Geometry: final body of the model. Coordinates: model frame, mm. A direction names the side the tool comes from. Give positions to 0.01 mm unless a question says otherwise; leave off trailing zeros. Loops run counter-clockwise (first coordinate to the right, second up) from the corner with the lowest first, then second, coordinate; pieces in that order, holes last. Notation, with made-up numbers: M 17,29 L 45,29 A32 ccw 45,57 Z; hole C 62,33.5 d11. An arc over 180 degrees is marked long. Put each result on its own line as item: value.
```python
from build123d import *

# Parameters (mm, degrees)
F1_DEPTH       = 25
F2_W           = 5
F2_H           = 25
F3_DEPTH       = 40
F4_R           = 5
F6_D           = 4
F6_CSINK_D     = 7
F6_CSINK_ANGLE = 90


# Not quite as in the source:
# - a feature names something its author has since deleted; it is built from what else it names


with BuildPart() as f1:
    # F0 (on Top) → F1 (new body)
    with BuildSketch(Plane.XY):
        with BuildLine():
            ThreePointArc((-14.3421743065, 17.5), (-10.0120472875, 16.123724357), (-7.2711064946, 12.5))
            Line((-7.2711064946, 12.5), (7.2711064946, 12.5))
            ThreePointArc((7.2711064946, 12.5), (10.0120472875, 16.123724357), (14.3421743065, 17.5))
            Line((14.3421743065, 17.5), (-14.3421743065, 17.5))
        make_face()
        with BuildLine():
            ThreePointArc((-7.2711064946, -12.5), (-10.0120472875, -16.123724357), (-14.3421743065, -17.5))
            Line((-14.3421743065, -17.5), (12.8716113806, -17.5))
            ThreePointArc((12.8716113806, -17.5), (8.5414843617, -16.123724357), (5.8005435687, -12.5))
            Line((5.8005435687, -12.5), (-7.2711064946, -12.5))
        make_face()
        with BuildLine():
            ThreePointArc((14.3421743065, 17.5), (10.0120472875, 16.123724357), (7.2711064946, 12.5))
            Line((7.2711064946, 12.5), (14.3421743065, 12.5))
            ThreePointArc((14.3421743065, 12.5), (16.1099412594, 11.767766953), (16.8421743065, 10))
            ThreePointArc((16.8421743065, 10), (16.1099412594, 8.232233047), (14.3421743065, 7.5))
            Line((14.3421743065, 7.5), (8.5, 7.5))
            ThreePointArc((8.5, 7.5), (12.7884854356, 6.1529580422), (15.5364989199, 2.5957047116))
            ThreePointArc((15.5364989199, 2.5957047116), (20.052140795, 5.1372556412), (21.8421743065, 10))
            ThreePointArc((21.8421743065, 10), (19.6454751654, 15.3033008589), (14.3421743065, 17.5))
        make_face()
        with BuildLine():
            ThreePointArc((-14.3421743065, 7.5), (-16.8421743065, 10), (-14.3421743065, 12.5))
            Line((-14.3421743065, 12.5), (-7.2711064946, 12.5))
            ThreePointArc((-7.2711064946, 12.5), (-10.0120472875, 16.123724357), (-14.3421743065, 17.5))
            ThreePointArc((-14.3421743065, 17.5), (-21.8182098422, 10.5990765131), (-15.5364989199, 2.5957047116))
            ThreePointArc((-15.5364989199, 2.5957047116), (-12.7884854356, 6.1529580422), (-8.5, 7.5))
            Line((-8.5, 7.5), (-14.3421743065, 7.5))
        make_face()
        with BuildLine():
            ThreePointArc((-7.3056753865, 7.4042952884), (-7.9009234869, 7.4760355357), (-8.5, 7.5))
            ThreePointArc((-8.5, 7.5), (-12.7884854356, 6.1529580422), (-15.5364989199, 2.5957047116))
            ThreePointArc((-15.5364989199, 2.5957047116), (-14.9412508196, 2.5239644643), (-14.3421743065, 2.5))
            ThreePointArc((-14.3421743065, 2.5), (-10.0536888708, 3.8470419578), (-7.3056753865, 7.4042952884))
        make_face()
        with BuildLine():
            ThreePointArc((-1, 0), (-2.7900335114, 4.8627443588), (-7.3056753865, 7.4042952884))
            ThreePointArc((-7.3056753865, 7.4042952884), (-10.0536888708, 3.8470419578), (-14.3421743065, 2.5))
            Line((-14.3421743065, 2.5), (-8.5, 2.5))
            ThreePointArc((-8.5, 2.5), (-6.732233047, 1.767766953), (-6, 0))
            ThreePointArc((-6, 0), (-6.732233047, -1.767766953), (-8.5, -2.5))
            Line((-8.5, -2.5), (-14.3421743065, -2.5))
            ThreePointArc((-14.3421743065, -2.5), (-10.0536888708, -3.8470419578), (-7.3056753865, -7.4042952884))
            ThreePointArc((-7.3056753865, -7.4042952884), (-2.7900335114, -4.8627443588), (-1, 0))
        make_face()
        with BuildLine():
            ThreePointArc((-14.3421743065, -2.5), (-14.9412508196, -2.5239644643), (-15.5364989199, -2.5957047116))
            ThreePointArc((-15.5364989199, -2.5957047116), (-12.7884854356, -6.1529580422), (-8.5, -7.5))
            ThreePointArc((-8.5, -7.5), (-7.9009234869, -7.4760355357), (-7.3056753865, -7.4042952884))
            ThreePointArc((-7.3056753865, -7.4042952884), (-10.0536888708, -3.8470419578), (-14.3421743065, -2.5))
        make_face()
        with BuildLine():
            ThreePointArc((12.8716113806, -2.5), (8.7359797123, -3.7432795568), (5.9714803927, -7.0609198123))
            ThreePointArc((5.9714803927, -7.0609198123), (7.2168200812, -7.3894146789), (8.5, -7.5))
            ThreePointArc((8.5, -7.5), (12.6356316683, -6.2567204432), (15.4001309879, -2.9390801877))
            ThreePointArc((15.4001309879, -2.9390801877), (14.1547912994, -2.6105853211), (12.8716113806, -2.5))
        make_face()
        with BuildLine():
            ThreePointArc((8.5, 7.5), (7.9009234869, 7.4760355357), (7.3056753865, 7.4042952884))
            ThreePointArc((7.3056753865, 7.4042952884), (9.8321935715, 4.0074985381), (13.7956134511, 2.5199417628))
            ThreePointArc((13.7956134511, 2.5199417628), (14.6682639838, 2.5070923186), (15.5364989199, 2.5957047116))
            ThreePointArc((15.5364989199, 2.5957047116), (12.7884854356, 6.1529580422), (8.5, 7.5))
        make_face()
        with BuildLine():
            ThreePointArc((13.7956134511, 2.5199417628), (9.8321935715, 4.0074985381), (7.3056753865, 7.4042952884))
            ThreePointArc((7.3056753865, 7.4042952884), (1.0317000428, 0.6888365189), (5.9714803927, -7.0609198123))
            ThreePointArc((5.9714803927, -7.0609198123), (8.7359797123, -3.7432795568), (12.8716113806, -2.5))
            Line((12.8716113806, -2.5), (8.5, -2.5))
            ThreePointArc((8.5, -2.5), (6.0000044235, -0.0047029402), (8.4905941362, 2.4999823059))
            Line((8.4905941362, 2.4999823059), (13.7956134511, 2.5199417628))
        make_face()
        with BuildLine():
            ThreePointArc((-8.5, -7.5), (-12.7884854356, -6.1529580422), (-15.5364989199, -2.5957047116))
            ThreePointArc((-15.5364989199, -2.5957047116), (-21.8182098422, -10.5990765131), (-14.3421743065, -17.5))
            ThreePointArc((-14.3421743065, -17.5), (-10.0120472875, -16.123724357), (-7.2711064946, -12.5))
            Line((-7.2711064946, -12.5), (-14.3421743065, -12.5))
            ThreePointArc((-14.3421743065, -12.5), (-16.8421743065, -10), (-14.3421743065, -7.5))
            Line((-14.3421743065, -7.5), (-8.5, -7.5))
        make_face()
        with BuildLine():
            Line((12.8716113806, -12.5), (5.8005435687, -12.5))
            ThreePointArc((5.8005435687, -12.5), (8.5414843617, -16.123724357), (12.8716113806, -17.5))
            ThreePointArc((12.8716113806, -17.5), (18.1749122395, -15.3033008589), (20.3716113806, -10))
            ThreePointArc((20.3716113806, -10), (19.0040618311, -5.6822399936), (15.4001309879, -2.9390801877))
            ThreePointArc((15.4001309879, -2.9390801877), (12.6356316683, -6.2567204432), (8.5, -7.5))
            Line((8.5, -7.5), (12.8716113806, -7.5))
            ThreePointArc((12.8716113806, -7.5), (14.6393783336, -8.232233047), (15.3716113806, -10))
            ThreePointArc((15.3716113806, -10), (14.6393783336, -11.767766953), (12.8716113806, -12.5))
        make_face()
    extrude(amount=F1_DEPTH)

    # F2 (on Right) → F3 (join, symmetric)
    with BuildSketch(Plane.YZ):
        with Locations((15, 12.5)):
            Rectangle(F2_W, F2_H)
    extrude(amount=F3_DEPTH, both=True)

    # F4
    f4_edges = [f1.edges().sort_by_distance(p)[0] for p in [
        (40, 15, 0),
        (40, 15, 25),
        (-40, 15, 25),
        (-40, 15, 0),
    ]]
    fillet(f4_edges, radius=F4_R)

    # F6 (through all)
    with Locations(Plane.XZ.offset(-12.5)):
        with Locations((27.5, 12.5), (-27.5, 12.5)):
            CounterSinkHole(F6_D / 2, F6_CSINK_D / 2, counter_sink_angle=F6_CSINK_ANGLE)


solid = f1.part
```
Item 1: Section D-D on z = 12.5. Count the separate pieces of the cut face and the enclosed holes in it, then the cut area to 3 significant figures.
Output values:
separate pieces: 3
enclosed holes: 1
area: 1,020 mm²
Item 2: Mould query, pull axis X, two halves, no side actions, for faces 5 (the cylindrical face through (-16.84, 9.95, 12.32)), 6 (the flat face through (-1, -17.5, 12)), 7 (the cylindrical face through (-39, 15, 2)). Classes: pulls with the +X half, pulls with the -X half, needs draft (parallel to the pull), parting line crosses it, or undercut.
Output values:
face 5: undercut
face 6: needs draft
face 7: pulls with the -X half
Item 3: Set-up query: faces 1 (the flat face through (-3, 0, 25)), 2 (the flat face through (11, -2.5, 12)), 3 (the flat face through (11, -7.5, 12)), 4 (the flat face through (-11, -2.5, 12)). Return all of +Z, -Z, +X, -X, +Y, -Y with unobstructed straight access to the full face (end or side cutting, diameter ignored); none if empty.
Output values:
face 1: +Z, +X, -X, +Y, -Y
face 2: +Z, -Z, +X
face 3: +Z, -Z
face 4: +Z, -Z, -X
Item 4: Section C-C on x = 4. Output: boundary loops of the cut face in (y, z).
Output values:
outline: M -17.5,0 L -12.5,0 L -12.5,25 L -17.5,25 Z; M -6,0 L 6,0 L 6,25 L -6,25 Z; M 12.5,0 L 17.5,0 L 17.5,25 L 12.5,25 Z
Item 5: Section B-B on y = -5. Output: boundary loops of the cut face in (x, z).
Output values:
outline: M -19.93,0 L -2.91,0 L -2.91,25 L -19.93,25 Z; M 2.91,0 L 18.46,0 L 18.46,25 L 2.91,25 Z
Item 6: Line query: probe 1 along X at (y, z) = (14.8, 12.5); probe 2 along Y at (x, z) = (-12.5, 9.25); probe 3 along X at (y, z) = (10, 7). Output: solid intervals per line, ascending. Write a range as [from, to].
Output values:
probe 1: [-40, -29.5], [-25.5, 25.5], [29.5, 40]
probe 2: [-17.5, -12.5], [-7.5, -2.5], [2.5, 7.5], [12.5, 17.5]
probe 3: [-21.84, -16.84], [16.84, 21.84]
Item 7: Section A-A on x = -12. Output: boundary loops of the cut face in (y, z), then the cut area to 3 significant figures.
Output values:
outline: M -17.5,0 L -12.5,0 L -12.5,25 L -17.5,25 Z; M -7.5,0 L -2.5,0 L -2.5,25 L -7.5,25 Z; M 2.5,0 L 7.5,0 L 7.5,25 L 2.5,25 Z; M 12.5,0 L 17.5,0 L 17.5,25 L 12.5,25 Z
area: 500 mm²
Item 8: Pin query (flat end, axial travel): pin 1 Ø5 at (y, z) = (1, 15) entering from +X; pin 2 Ø6 at (y, z) = (-4, 12) entering from +X; pin 3 Ø2 at (x, y) = (8, -3) entering from -Z; pin 4 Ø8 at (x, z) = (25, 19) entering from -Y. Return the tip coordinate at first contact, or that it passes through.
Output values:
pin 1: x = 18.08
pin 2: x = 19.75
pin 3: z = 0
pin 4: y = 6.55
